Autodesk Inventor part; units mm, degrees
ref_plane "YZ Plane" through (0, 0, 0) normal (1, 0, 0) x (0, 1, 0)
ref_plane "XZ Plane" through (0, 0, 0) normal (0, 1, 0) x (-1, 0, 0)
ref_plane "XY Plane" through (0, 0, 0) normal (0, 0, 1) x (1, 0, 0)
sketch "Sketch1" plane through (0, 0, 0) normal (0, 0, 1) x (1, 0, 0)
  line L0 (-12.7, 0) -> (12.7, 0)
  line L1 (-12.7, 0) -> (-12.7, 25.4)
  line L2 (12.7, 0) -> (12.7, 25.4)
  line L3 (-9.525, 25.4) -> (-9.525, 3.175)
  line L4 (-9.525, 3.175) -> (9.525, 3.175)
  line L5 (9.525, 3.175) -> (9.525, 25.4)
  line L6 (-12.7, 25.4) -> (-9.525, 25.4)
  line L7 (9.525, 25.4) -> (12.7, 25.4)
  point P0 (0, 0)
  point P1 (0, 0)
  dimension "d0" = 25.4
  dimension "d1" = 25.4
  dimension "d2" = 25.4
  dimension "d3" = 3.175
extrude "Extrusion1" add sketch "Sketch1" along normal blind 120
sketch "Sketch2" plane through (-9.525, 3.175, 0) normal (0, 1, 0) x (1, 0, 0)
  circle A0 centre (9.525, -11) radius 2.1
  line L0 (-3.175, 0) -> (-3.175, -120) construction
  circle A1 centre (9.525, -25) radius 2.1
  circle A2 centre (9.525, -39) radius 2.1
  circle A3 centre (9.525, -53) radius 2.1
  circle A4 centre (9.525, -67) radius 2.1
  circle A5 centre (9.525, -81) radius 2.1
  circle A6 centre (9.525, -95) radius 2.1
  circle A7 centre (9.525, -109) radius 2.1
  line L1 (9.525, -67) -> (9.525, -53) construction
  line L2 (19.05, 0) -> (19.05, -120)
  line L3 (19.05, 0) -> (0, 0)
  point P0 (9.525, 0)
  point P1 (9.525, -60)
  point P2 (19.05, -60)
  point P3 (9.525, 0)
  dimension "d6" = 4.2
  dimension "d10" = 14
extrude "Extrusion2" cut sketch "Sketch2" against normal through all
sketch "Sketch3" plane through (12.7, 0, 0) normal (1, 0, 0) x (0, 0, -1)
  circle A0 centre (-11, 15.875) radius 2.1
  line L0 (0, 3.175) -> (0, 25.4) construction
  line L1 (0, 25.4) -> (-120, 25.4) construction
  circle A1 centre (-25, 15.875) radius 2.1
  circle A2 centre (-39, 15.875) radius 2.1
  circle A3 centre (-53, 15.875) radius 2.1
  circle A4 centre (-67, 15.875) radius 2.1
  circle A5 centre (-81, 15.875) radius 2.1
  circle A6 centre (-95, 15.875) radius 2.1
  circle A7 centre (-109, 15.875) radius 2.1
  line L2 (-67, 15.875) -> (-53, 15.875) construction
  line L3 (0, 0) -> (-120, 0)
  point P0 (-60, 15.875)
  point P1 (-60, 25.4)
  dimension "d17" = 4.2
  dimension "d21" = 14
  dimension "d35" = 15.875
extrude "Extrusion3" cut sketch "Sketch3" against normal through all
hole "Hole1" at (0, 3.175, 109) at (0, 3.175, 95) at (0, 3.175, 81) at (0, 3.175, 67) at (0, 3.175, 53) at (0, 3.175, 39) at (0, 3.175, 25) at (0, 3.175, 11) direction (0, -1, 0) diameter 4.2 end through all countersink diameter 8 countersink angle 90
properties part number "C-Channel_ArmSupport"
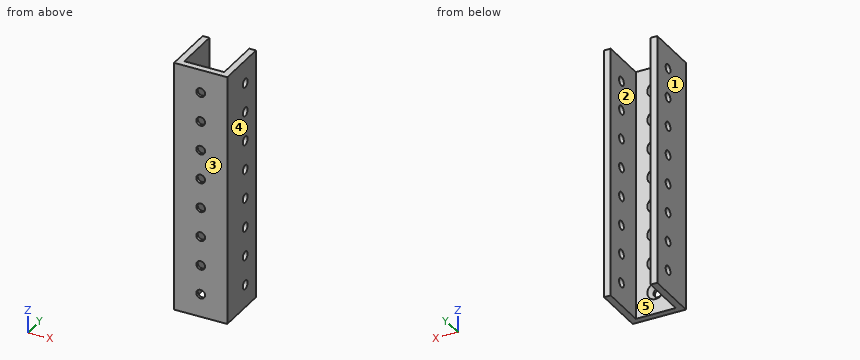
Here's how the part is built. I have some questions about the finished solid (model axes, mm). Face numbers are marked on the shaded views. A direction names the side the tool comes from. Coordinates: 2 decimals unless noted, no trailing zeros. Write each loop counter-clockwise with the first axis right and the second up, starting at its lowest first coordinate (ties: lowest second). Pieces come first, ordered by that corner, then holes. Notation, with made-up numbers: (50, 87.5) - (87, 87.5) arc R14 ccw to (87, 104.5) - close; hole circle Ø4 at (-16, 55). An arc over 180 degrees is marked (long way). Use one line per item in the form item = value.
1) Thinking about a two-plate mould opening in X: for the marked faces 3, 4 and 5, which applies, released by +X, released by -X, zero draft, split by the parting line, or undercut?
Solved:
face_3 = zero draft
face_4 = released by +X
face_5 = undercut
2) I need wall thicknesses on line 1 (X direction, y = 16.75, z = 21) (3 decimals); line 2 (Y direction, x = -10.7, z = 11) (3 decimals); line 3 (Y direction, x = -4, z = 21.5) (3 decimals). Which ranges of each line are inside material? Lowest first, please.
Solved:
line_1 = -12.7 to -9.525, 9.525 to 12.7
line_2 = 0 to 13.775, 17.975 to 25.4
line_3 = 0 to 3.175
3) Suppose I cut it at C-C, the plane x = 0. Give the number of separate pieces and of enclosed holes in the cut face, plus the area to 3 significant figures.
Solved:
separate_pieces = 9
enclosed_holes = 0
area = 245 mm2
4) Suppose I cut it at A-A, the plane y = 5. Write out the boundary of the cut face in (x, z) (3 decimals).
Solved:
outline = (-12.7, 0) - (-9.525, 0) - (-9.525, 120) - (-12.7, 120) - close; (9.525, 0) - (12.7, 0) - (12.7, 120) - (9.525, 120) - close
5) Suppose I cut it at B-B, the plane z = 11. Write out the boundary of the cut face in (x, y) (3 decimals).
Solved:
outline = (-12.7, 0) - (-2.1, 0) - (-2.1, 1.275) - (-4, 3.175) - (-9.525, 3.175) - (-9.525, 13.775) - (-12.7, 13.775) - close; (-12.7, 17.975) - (-9.525, 17.975) - (-9.525, 25.4) - (-12.7, 25.4) - close; (2.1, 0) - (12.7, 0) - (12.7, 13.775) - (9.525, 13.775) - (9.525, 3.175) - (4, 3.175) - (2.1, 1.275) - close; (9.525, 17.975) - (12.7, 17.975) - (12.7, 25.4) - (9.525, 25.4) - close
6) I'm going to push flat-ended pins straight in: P1, Ø6.5, axis at x = 0, z = 95, coming from the -Y side; P2, Ø5.5, axis at x = -2.5, z = 77.5, coming from the +Y side (3 decimals). Where does each tip first touch, or does it pass through?
Solved:
P1 = 0
P2 = 3.175
7) Suppose I cut it at D-D, the plane x = -6. Write out the boundary of the cut face in (y, z) (3 decimals).
Solved:
outline = (0, 0) - (3.175, 0) - (3.175, 120) - (0, 120) - close
8) On a 3-axis mill with a long thin cutter (end or side, diameter ignored), from which of +Z, -Z, +X, -X, +Y, -Y can I reach the whole of each face in a straight line? I mean the marked faces 1 and 2. Say none if no direction works.
Solved:
face_1 = +Z, -Z, -X, +Y, -Y
face_2 = +Z, -Z, +Y
